For this review, take the finished solid that the model builds, in its own axes (mm). A direction names the side the tool comes from. Give positions to 0.01 mm unless a question says otherwise; leave off trailing zeros. Write each loop counter-clockwise with the first axis right and the second up, starting at its lowest first coordinate (ties: lowest second). Pieces come first, ordered by that corner, then holes. Notation, with made-up numbers: M 47.25,88.5 L 100.25,88.5 A27 cw 100.25,110.5 Z; hole C 25.25,13 d8. An arc over 180 degrees is marked long. Use one line per item in the form item = value. Start each with the question number.
Q1. Tool access review of faces 4 (the cylindrical face through (-0.34, -2.44, -0.54)), 5 (the flat face through (-6.254, 2.7, -4.4)): name each direction out of +Z, -Z, +X, -X, +Y, -Y from which nothing blocks a thin tool from reaching the whole face with its end or side.
Q2. For probe 1 along Y at (x, z) = (-3.5, 0); probe 2 along X at (y, z) = (-0.25, 3.75); probe 3 along Y at (x, z) = (3.75, -0.25), list the stretches that pass through material, from the lowest coordinate up. Write a range as [from, to].
Q3. Consider section A-A on z = 0. Write out the cut boundary in (x, y), and give its area (3 significant figures).
Q4. Consider section D-D on z = -4.5. Write out the cut boundary in (x, y), and give its area (3 significant figures).
Q5. Mouldability with a two-part tool opening along Z and no side actions: class faces 1 (the cylindrical face through (3.303, 4.141, -0.587)), 2 (the cylindrical face through (-6.73, -3.59, -4.69)), 3 (the flat face through (6.7, -1.08, -2.45)) as released by +Z, released by -Z, zero draft, split by the parting line, or undercut.
Q6. Clearance check with flat-ended pins moving along their axes: pin 1 Ø3 at (x, y) = (-2, 1) entering from -Z; pin 2 Ø3 at (y, z) = (0, 0) entering from +X; pin 3 Ø5 at (x, y) = (0, 3.5) entering from +Z; pin 4 Ø1 at (x, z) = (-4.5, -1) entering from +Y. State where each tip first meets the part, or that it passes through.
Q7. Consider section C-C on x = -2.25. Write out the cut boundary in (y, z), and give its area (3 significant figures).
```python
from build123d import *

# Parameters (mm, degrees)
BASPROSKE_W         = 6.7
BASPROSKE_H         = 4.9
TOOTHCUT_DEPTH      = 10.638983349
TEETHCUTS_COUNT     = 12
TEETHCUTS_ANGLE     = 330
BORSKE_R            = 0.4
BORE_DEPTH          = 50.0000508
SKETCH1_R           = 5
BOSS_EXTRUDE1_DEPTH = 7.1938
SKETCH3_R           = 5.9055
BOSS_EXTRUDE2_DEPTH = 0.9398
SKETCH2_R           = 2.5
CUT_EXTRUDE1_DEPTH  = 17.210722962


with BuildPart() as part:
    # BasProSke → Base-Revolve (revolve)
    with BuildSketch(Plane(origin=(0, 0, 0), x_dir=(1, 0, 0), z_dir=(0, 1, 0)), mode=Mode.PRIVATE) as base_revolve_sk:
        with Locations((3.35, 2.45)):
            Rectangle(BASPROSKE_W, BASPROSKE_H)
    revolve(base_revolve_sk.sketch.rotate(Axis((-10, 0, 0), (1, 0, 0)), 180), axis=Axis((-10, 0, 0), (1, 0, 0)))

    # TooCutSke → ToothCut (cut, through all)
    with BuildSketch(Plane(origin=(0, 0, 0), x_dir=(0, 0, -1), z_dir=(1, 0, 0))):
        with BuildLine():
            ThreePointArc((0.394109641, 3.300553528), (0, 3.324), (-0.394109641, 3.300553528))
            ThreePointArc((-0.394109641, 3.300553528), (-0.589367544, 4.146348526), (-1.180740601, 4.781779668))
            ThreePointArc((-1.180740601, 4.781779668), (0, 4.9254), (1.180740601, 4.781779668))
            ThreePointArc((1.180740601, 4.781779668), (0.589367544, 4.146348526), (0.394109641, 3.300553528))
        make_face()
    toothcut = extrude(amount=TOOTHCUT_DEPTH, mode=Mode.SUBTRACT)

    # TeethCuts: ToothCut ×12 about axis
    teethcuts_axis = Axis((-10, 0, 0), (1, 0, 0))
    for i in range(1, TEETHCUTS_COUNT):
        add(toothcut.rotate(teethcuts_axis, i * TEETHCUTS_ANGLE / (TEETHCUTS_COUNT - 1)), mode=Mode.SUBTRACT)

    # BorSke → Bore (cut, symmetric)
    with BuildSketch(Plane(origin=(0, 0, 0), x_dir=(0, 0, -1), z_dir=(1, 0, 0))):
        with Locations(Location((0, 0, 0), (0, 0, 180))):
            Circle(BORSKE_R)
    extrude(amount=BORE_DEPTH, both=True, mode=Mode.SUBTRACT)

    # Sketch1 → Boss-Extrude1 (add)
    with BuildSketch(Plane.ZY):
        Circle(SKETCH1_R)
    extrude(amount=BOSS_EXTRUDE1_DEPTH)

    # Sketch3 → Boss-Extrude2 (add)
    with BuildSketch(Plane.ZY.offset(7.1938)):
        Circle(SKETCH3_R)
    extrude(amount=-BOSS_EXTRUDE2_DEPTH)

    # Sketch2 → Cut-Extrude1 (cut, through all)
    with BuildSketch(Plane.ZY.offset(7.1938)):
        Circle(SKETCH2_R)
    extrude(amount=-CUT_EXTRUDE1_DEPTH, mode=Mode.SUBTRACT)


solid = part.part
```
Working result:
q1.face_4 = +X, -X
q1.face_5 = +X
q2.probe_1 = [-5, -2.5], [2.5, 5]
q2.probe_2 = [-7.19, 0]
q2.probe_3 = [-3.31, -2.49], [2.49, 3.31]
q3.outline = M -7.19,-5.91 L -6.25,-5.91 L -6.25,-5 L 0,-5 L 0,-3.32 L 6.7,-3.32 L 6.7,-2.5 L -7.19,-2.5 Z; M -7.19,2.5 L 6.7,2.5 L 6.7,3.32 L 0,3.32 L 0,5 L -6.25,5 L -6.25,5.91 L -7.19,5.91 Z
q3.area = 48.7 mm²
q4.outline = M -7.19,-3.82 L -6.25,-3.82 L -6.25,-2.18 L 0,-2.18 L 0,-1.47 L 6.7,-1.47 L 6.7,-0.84 L 0,-0.84 L 0,0.84 L 6.7,0.84 L 6.7,1.47 L 0,1.47 L 0,2.18 L -6.25,2.18 L -6.25,3.82 L -7.19,3.82 Z
q4.area = 42.9 mm²
q5.face_1 = undercut
q5.face_2 = split by the parting line
q5.face_3 = zero draft
q6.pin_1 = -5
q6.pin_2 = through
q6.pin_3 = 4.9
q6.pin_4 = 4.97
q7.outline = C 0,0 d10; hole C 0,0 d5
q7.area = 58.9 mm²
